Verification items for the finished model (mm, model axes). A direction names the side the tool comes from. Round coordinates to 2 decimals unless told otherwise and drop trailing zeros. Order: outer loops, then holes, each group sorted by start corner. A loop starts at its lowest first (then second) coordinate and runs counter-clockwise, first axis right, second up. Notation, with made-up numbers: M 16.5,-6 L 47.5,-6 A23 cw 47.5,21 Z; hole C 76,63 d7. An arc over 180 degrees is marked long. Return JSON: item names as keys, results as strings. Group by question number.
from build123d import *

# Parameters (mm, degrees)
SKETCH_W     = 44
SKETCH_H     = 89
PAD_DEPTH    = 10
PAD001_DEPTH = 7
PAD002_DEPTH = 7


with BuildPart() as part:
    # Sketch → Pad (new body)
    with BuildSketch(Plane.XY):
        Polygon((-22, 0), (-18, 0), (-18, -5), (18, -5), (18, 0), (22, 0), (22, 4), (27, 4), (27, 15), (22, 15), (22, 19), (21.5, 19), (21.5, 20), (29, 20), (29, -100), (-29, -100), (-29, 20), (-21.5, 20), (-21.5, 19), (-22, 19), (-22, 15), (-27, 15), (-27, 4), (-22, 4), align=None)
        with Locations((0, -53.5)):
            Rectangle(SKETCH_W, SKETCH_H, mode=Mode.SUBTRACT)
    extrude(amount=PAD_DEPTH)

    # Sketch001 (on DatumPlane) → Pad001 (join)
    with BuildSketch(Plane.YZ.offset(-22)):
        with BuildLine():
            Line((-100, 0), (-100, 30))
            Line((-95, 30), (-100, 30))
            ThreePointArc((-95, 30), (-88.049566, 10.375362), (-70, 0))
            Line((-100, 0), (-70, 0))
        make_face()
    extrude(amount=-PAD001_DEPTH)

    # Sketch002 (on DatumPlane) → Pad002 (join)
    with BuildSketch(Plane.YZ.offset(22)):
        with BuildLine():
            Line((-100, 0), (-100, 30))
            Line((-95, 30), (-100, 30))
            ThreePointArc((-95, 30), (-88.049566, 10.375362), (-70, 0))
            Line((-100, 0), (-70, 0))
        make_face()
    extrude(amount=PAD002_DEPTH)


solid = part.part
1. Cross-section at A-A (y = -83). Enter the section's corners in (x, z).
2. Cross-section at B-B (z = 3.25). Enter the section's corners in (x, y), plus the area to 4 significant figures.
3. Cross-section at C-C (x = 16). Enter the section's corners in (y, z), plus the area to 3 significant figures.
4. Draft check along X on faces 4 (the face through (29, -44, 6)), 5 (the face through (24, -34, 10)), 6 (the face through (-24, 15, 5)). Enter one of: +X half, -X half, draft (parallel to the pull), parting line (faces both ways), or undercut.
5. Access from +Z, -Z, +X, -X, +Y, -Y to the whole of each face (thin tool, end or side, straight path). Record for faces 1 (the face through (-25, 20, 5)), 2 (the face through (-22, 2, 5)), 3 (the face through (0, -5, 5)).
6. Go/stop test with flat-tipped pins: pin 1 (1.2 mm diameter, centred on x = 20.5, z = 4, fed in from +Y); pin 2 (3 mm diameter, centred on x = 1.5, z = 4, fed in from +Y); pin 3 (3 mm diameter, centred on x = -20, z = 16, fed in from +Y). Record where each tip stops, or that it passes through.
7. Thickness scan on line 1 along X through (y, z) = (-74, 6.75); line 2 along Y through (x, z) = (16.5, 4.75); line 3 along X through (y, z) = (12, 7). Record the ranges inside material, lowest first. Write a range as from..to.
Computed:
{
 "1": {"outline": "M -29,0 L -22,0 L -22,10 L -29,10 Z; M 22,0 L 29,0 L 29,10 L 22,10 Z"},
 "2": {"outline": "M -29,-100 L 29,-100 L 29,20 L 21.5,20 L 21.5,19 L 22,19 L 22,15 L 27,15 L 27,4 L 22,4 L 22,0 L 18,0 L 18,-5 L -18,-5 L -18,0 L -22,0 L -22,4 L -27,4 L -27,15 L -22,15 L -22,19 L -21.5,19 L -21.5,20 L -29,20 Z; hole M -22,-98 L 22,-98 L 22,-9 L -22,-9 Z", "area": "1,875 mm²"},
 "3": {"outline": "M -100,0 L -98,0 L -98,10 L -100,10 Z; M -9,0 L -5,0 L -5,10 L -9,10 Z", "area": "60.0 mm²"},
 "4": {"face 4": "+X half", "face 5": "draft", "face 6": "undercut"},
 "5": {"face 1": "+Z, -Z, +X, -X, +Y", "face 2": "+Z, -Z", "face 3": "+Z, -Z, +Y"},
 "6": {"pin 1": "stops at y = 0", "pin 2": "stops at y = -5", "pin 3": "passes through"},
 "7": {"line 1": "x = -29..-22, 22..29", "line 2": "y = -100..-98, -9..-5", "line 3": "x = -29..-27, 27..29"}
}
